```python
from build123d import *

# Parameters (mm, degrees)
SKETCH_1_R          = 1.6
EXTRUDE_1_DEPTH     = 2
SKETCH_2_R          = 10.85
EXTRUDE_2_DEPTH     = 3
EXTRUDE_3_DEPTH     = 8
SKETCH_4_R          = 9.9
EXTRUDE_4_DEPTH     = 10
CHAMFER_1_SIZE      = 1
CHAMFER_2_SIZE      = 1
SKETCH_5_R          = 10
SKETCH_5_R_2        = 1
CUT_EXTRUDE_1_DEPTH = 10


with BuildPart() as part:
    # 草图1 → 凸台-拉伸1 (new body)
    with BuildSketch(Plane.XY):
        with BuildLine():
            Line((-11.5, -14.5), (11.5, -14.5))
            ThreePointArc((11.5, -14.5), (13.621320344, -13.621320344), (14.5, -11.5))
            Line((14.5, -11.5), (14.5, 11.5))
            ThreePointArc((14.5, 11.5), (13.621320344, 13.621320344), (11.5, 14.5))
            Line((11.5, 14.5), (-11.5, 14.5))
            ThreePointArc((-11.5, 14.5), (-13.621320344, 13.621320344), (-14.5, 11.5))
            Line((-14.5, 11.5), (-14.5, -11.5))
            ThreePointArc((-14.5, -11.5), (-13.621320344, -13.621320344), (-11.5, -14.5))
        make_face()
        with Locations((11, 11)):
            Circle(SKETCH_1_R, mode=Mode.SUBTRACT)
        with Locations(Location((-11, 11, 0), (0, 0, 180))):
            Circle(SKETCH_1_R, mode=Mode.SUBTRACT)
        with Locations((-11, -11)):
            Circle(SKETCH_1_R, mode=Mode.SUBTRACT)
        with Locations(Location((11, -11, 0), (0, 0, 180))):
            Circle(SKETCH_1_R, mode=Mode.SUBTRACT)
    extrude(amount=-EXTRUDE_1_DEPTH)

    # 草图2 → 凸台-拉伸2 (add)
    with BuildSketch(Plane.XY):
        with Locations(Location((0, 0, 0), (0, 0, 180))):
            Circle(SKETCH_2_R)
    extrude(amount=EXTRUDE_2_DEPTH)

    # 草图3 → 凸台-拉伸3 (add)
    with BuildSketch(Plane.XY.offset(3)):
        with BuildLine():
            Line((13.374827304, 1.834119567), (8.275807791, 10.665880433))
            ThreePointArc((8.275807791, 10.665880433), (6.75, 11.691342951), (5.099019514, 12.5))
            Line((5.099019514, 12.5), (-5.099019514, 12.5))
            ThreePointArc((-5.099019514, 12.5), (-6.75, 11.691342951), (-8.275807791, 10.665880433))
            Line((-8.275807791, 10.665880433), (-13.374827304, 1.834119567))
            ThreePointArc((-13.374827304, 1.834119567), (-13.5, 0), (-13.374827304, -1.834119567))
            Line((-13.374827304, -1.834119567), (-8.275807791, -10.665880433))
            ThreePointArc((-8.275807791, -10.665880433), (-6.75, -11.691342951), (-5.099019514, -12.5))
            Line((-5.099019514, -12.5), (5.099019514, -12.5))
            ThreePointArc((5.099019514, -12.5), (6.75, -11.691342951), (8.275807791, -10.665880433))
            Line((8.275807791, -10.665880433), (13.374827304, -1.834119567))
            ThreePointArc((13.374827304, -1.834119567), (13.5, 0), (13.374827304, 1.834119567))
        make_face()
    extrude(amount=EXTRUDE_3_DEPTH)

    # 草图4 → 凸台-拉伸4 (add)
    with BuildSketch(Plane(origin=(0, 0, -2), x_dir=(-1, 0, 0), z_dir=(0, 0, -1))):
        Circle(SKETCH_4_R)
    extrude(amount=EXTRUDE_4_DEPTH)

    # 倒角1
    chamfer_1_edges = [part.edges().sort_by_distance(p)[0] for p in [
        (-6.75, -11.691342951, 3),
        (-13.5, 0, 3),
        (-6.75, 11.691342951, 3),
        (6.75, 11.691342951, 3),
        (6.75, -11.691342951, 3),
        (13.5, 0, 3),
    ]]
    chamfer(chamfer_1_edges, length=CHAMFER_1_SIZE - 0.0001)  # a hair under: the kernel refuses the full size

    # 倒角2
    chamfer_2_edges = [part.edges().sort_by_distance(p)[0] for p in [
        (13.5, 0, 11),
        (6.75, 11.691342951, 11),
        (6.75, -11.691342951, 11),
        (-6.75, -11.691342951, 11),
        (-6.75, 11.691342951, 11),
        (-13.5, 0, 11),
    ]]
    chamfer(chamfer_2_edges, length=CHAMFER_2_SIZE - 0.0001)  # a hair under: the kernel refuses the full size

    # 草图5 → 切除-拉伸1 (cut)
    with BuildSketch(Plane.XY.offset(11)):
        Circle(SKETCH_5_R)
        with Locations((-3.66926495, 7.697601599)):
            Circle(SKETCH_5_R_2, mode=Mode.SUBTRACT)
        with Locations((3.593463585, 7.697601599)):
            Circle(SKETCH_5_R_2, mode=Mode.SUBTRACT)
        with Locations((-7.680655711, 3.179508847)):
            Circle(SKETCH_5_R_2, mode=Mode.SUBTRACT)
        with Locations((0, 3.179508847)):
            Circle(SKETCH_5_R_2, mode=Mode.SUBTRACT)
        with Locations((7.309278185, 3.179508847)):
            Circle(SKETCH_5_R_2, mode=Mode.SUBTRACT)
        with Locations((-4.63214688, -0.87410708)):
            Circle(SKETCH_5_R_2, mode=Mode.SUBTRACT)
        with Locations((3.889039747, -0.87410708)):
            Circle(SKETCH_5_R_2, mode=Mode.SUBTRACT)
        with Locations((-4.63214688, -5.3077495)):
            Circle(SKETCH_5_R_2, mode=Mode.SUBTRACT)
        with Locations((3.889039747, -4.969948172)):
            Circle(SKETCH_5_R_2, mode=Mode.SUBTRACT)
    extrude(amount=-CUT_EXTRUDE_1_DEPTH, mode=Mode.SUBTRACT)


solid = part.part
```
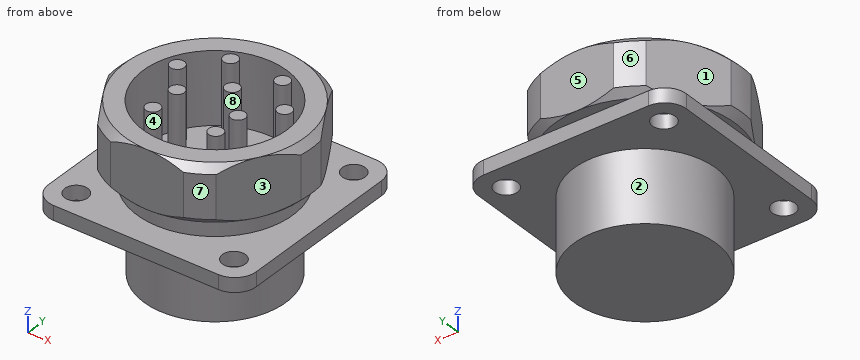
Part model, mm, in its own coordinate system. Face numbers are marked on the shaded views. A direction names the side the tool comes from. Coordinates: 2 decimals unless noted, no trailing zeros. Write each loop counter-clockwise with the first axis right and the second up, starting at its lowest first coordinate (ties: lowest second). Pieces come first, ordered by that corner, then holes.
Item 1: Pin check, flat tips, straight feed: pin 1 (8 mm diameter, centred on x = -5.5, y = 11.5, fed in from +Z); pin 2 (3 mm diameter, centred on y = -9, z = 2.5, fed in from +X); pin 3 (6.5 mm diameter, centred on x = -1, z = 7.5, fed in from -Y); pin 4 (1 mm diameter, centred on y = 7.5, z = -5, fed in from +X). Stop position of each tip, or through.
Item 2: Slice it at B-B (z = -5.5). Write the cut outline in (x, y), and give its area (3 significant figures).
Item 3: Mould opens along Y. For the marked faces 6, 7 and 8 say: released by +Y, released by -Y, zero draft, split by the parting line, or undercut.
Item 4: Slice it at A-A (z = 5.75). Count the separate pieces of the cut face and the enclosed holes in it, and give its area (3 significant figures).
Item 5: Probe line 1 (Y direction, x = -11, z = -1.4); line 2 (Z direction, x = 10.5, y = 5.5); line 3 (Y direction, x = 0.25, z = 2). List the from-to ranges inside material, lowest first.
Item 6: Which spindle directions (+Z, -Z, +X, -X, +Y, -Y) get a long thin tool onto all of the face, cutting with end or side? Do the marked faces 1, 2, 3, 4 and 5. Say none if no direction does.
Results found:
1. pin 1: stops at z = 11
1. pin 2: stops at x = 10.03
1. pin 3: stops at y = -12.5
1. pin 4: stops at x = 7
2. outline: circle Ø19.8 at (0, 0)
2. area: 308 mm2
3. face 6: released by +Y
3. face 7: released by -Y
3. face 8: undercut
4. separate pieces: 10
4. enclosed holes: 1
4. area: 246 mm2
5. line 1: y = -14.5 to -12.6, -9.4 to 9.4, 12.6 to 14.5
5. line 2: z = -2 to 0, 3 to 11
5. line 3: y = -10.85 to -10, 2.21 to 4.15, 10 to 10.85
6. face 1: +Z, -X, +Y
6. face 2: -Z
6. face 3: +Z, +X, -Y
6. face 4: +Z
6. face 5: +Z, +X, -X, +Y
